CAD build for the part. Positions are in the model's coordinates, mm. Round coordinates to 2 decimals unless told otherwise and drop trailing zeros. Write each loop counter-clockwise with the first axis right and the second up, starting at its lowest first coordinate (ties: lowest second). Pieces come first, ordered by that corner, then holes. Notation, with made-up numbers: M 56,28 L 78,28 A28 cw 78,59 Z; hole C 58,75 d3. An arc over 180 degrees is marked long. Write each question's results on one line, items separated by ' | '. Start each with the question number.
```python
from build123d import *

# Parameters (mm, degrees)
CROQUIS1_W                  = 215.9
CROQUIS1_H                  = 146.05
SALIENTE_EXTRUIR1_DEPTH     = 3.1242
CROQUIS2_R                  = 1.3335
CORTAR_EXTRUIR1_DEPTH       = 131.36722652
CROQUIS9_R                  = 1.27
CORTAR_EXTRUIR6_DEPTH       = 131.36722652
CORTAR_EXTRUIR2_DEPTH       = 131.36722652
DIFERENCIAL_TRASERO_DEPTH   = 131.36722652
ENTRADA_TRANSMISION_DEPTH   = 131.36722652
CROQUIS10_R                 = 1.016
CROQUIS10_W                 = 22.606
CROQUIS10_H                 = 11.9888
CROQUIS10_W_2               = 2.032
CROQUIS10_H_2               = 5.08
SERVO_DEPTH                 = 131.36722652
CROQUIS12_R                 = 1.651
SOPORTES_BS_DEPTH           = 131.36722652
CROQUIS7_R                  = 1.5875
CROQUIS7_W                  = 11.1125
CROQUIS7_H                  = 2.9972
SOPORTE_EJE_DEPTH           = 131.36722652
CROQUIS13_R                 = 1.016
CROQUIS13_W                 = 10.922
CROQUIS13_H                 = 2.9972
CROQUIS13_W_2               = 2.9972
CROQUIS13_H_2               = 10.922
SENSORES_DE_PRESENCIA_DEPTH = 131.36722652


with BuildPart() as part:
    # Croquis1 → Saliente-Extruir1 (new body)
    with BuildSketch(Plane.XY):
        Rectangle(CROQUIS1_W, CROQUIS1_H)
    extrude(amount=SALIENTE_EXTRUIR1_DEPTH)

    # Croquis2 → Cortar-Extruir1 (cut, through all)
    with BuildSketch(Plane.XY.offset(3.1242)):
        with BuildLine():
            ThreePointArc((82.1674125, 60.7314), (81.516352882, 61.877042778), (80.1989125, 61.904002767))
            Line((80.1989125, 61.904002767), (80.1989125, 59.558797233))
            ThreePointArc((80.1989125, 59.558797233), (81.516352882, 59.585757222), (82.1674125, 60.7314))
        make_face()
        with BuildLine():
            Line((80.1989125, 59.558797233), (80.1989125, 61.904002767))
            ThreePointArc((80.1989125, 61.904002767), (79.5004125, 60.7314), (80.1989125, 59.558797233))
        make_face()
        with Locations(Location((80.8339125, -60.7314, 0), (0, 0, 180))):
            Circle(CROQUIS2_R)
    extrude(amount=-CORTAR_EXTRUIR1_DEPTH, mode=Mode.SUBTRACT)

    # Croquis9 → Cortar-Extruir6 (cut, through all)
    with BuildSketch(Plane.XY.offset(3.1242)):
        with Locations((93.5339125, 37.6809)):
            Circle(CROQUIS9_R)
        with Locations(Location((93.5339125, -37.6809, 0), (0, 0, 180))):
            Circle(CROQUIS9_R)
        with Locations((79.5639125, 37.6809)):
            Circle(CROQUIS9_R)
        with Locations((79.5639125, -37.6809)):
            Circle(CROQUIS9_R)
    extrude(amount=-CORTAR_EXTRUIR6_DEPTH, mode=Mode.SUBTRACT)

    # Croquis3 → Cortar-Extruir2 (cut, through all)
    with BuildSketch(Plane.XY.offset(3.1242)):
        with BuildLine():
            ThreePointArc((31.75, 73.025), (36.240128061, 71.165128061), (38.1, 66.675))
            Line((38.1, 66.675), (38.1, 60.648925294))
            ThreePointArc((38.1, 60.648925294), (44.483976367, 49.058906773), (56.88726875, 44.45))
            ThreePointArc((56.88726875, 44.45), (68.952768587, 48.752886462), (75.572740263, 59.719521917))
            ThreePointArc((75.572740263, 59.719521917), (75.649024122, 60.222907145), (75.6745375, 60.7314))
            ThreePointArc((75.6745375, 60.7314), (79.079726884, 65.583408163), (84.800442563, 64.030762007))
            ThreePointArc((84.800442563, 64.030762007), (101.984927744, 34.043503392), (107.95, 0))
            Line((107.95, 0), (107.95, 73.025))
            Line((107.95, 73.025), (31.75, 73.025))
        make_face()
        with BuildLine():
            Line((107.95, -73.025), (107.95, 0))
            ThreePointArc((107.95, 0), (101.984927744, -34.043503392), (84.800442563, -64.030762007))
            ThreePointArc((84.800442563, -64.030762007), (79.079726884, -65.583408163), (75.6745375, -60.7314))
            ThreePointArc((75.6745375, -60.7314), (75.649024122, -60.222907145), (75.572740263, -59.719521917))
            ThreePointArc((75.572740263, -59.719521917), (68.952768587, -48.752886462), (56.88726875, -44.45))
            ThreePointArc((56.88726875, -44.45), (44.483976367, -49.058906773), (38.1, -60.648925294))
            Line((38.1, -60.648925294), (38.1, -66.675))
            ThreePointArc((38.1, -66.675), (36.240128061, -71.165128061), (31.75, -73.025))
            Line((31.75, -73.025), (107.95, -73.025))
        make_face()
        with BuildLine():
            ThreePointArc((-107.95, 63.5), (-105.160192091, 70.235192091), (-98.425, 73.025))
            Line((-98.425, 73.025), (-107.95, 73.025))
            Line((-107.95, 73.025), (-107.95, 63.5))
        make_face()
        with BuildLine():
            Line((-107.95, -73.025), (-98.425, -73.025))
            ThreePointArc((-98.425, -73.025), (-105.160192091, -70.235192091), (-107.95, -63.5))
            Line((-107.95, -63.5), (-107.95, -73.025))
        make_face()
    extrude(amount=-CORTAR_EXTRUIR2_DEPTH, mode=Mode.SUBTRACT)

    # Croquis8 → Diferencial trasero (cut, through all)
    with BuildSketch(Plane.XY.offset(3.1242)):
        with BuildLine():
            Line((-62.484, 29.2862), (-59.944, 29.2862))
            ThreePointArc((-59.944, 29.2862), (-58.674, 28.0162), (-59.944, 26.7462))
            Line((-59.944, 26.7462), (-62.484, 26.7462))
            ThreePointArc((-62.484, 26.7462), (-63.754, 28.0162), (-62.484, 29.2862))
        make_face()
        with BuildLine():
            Line((-95.25, 55.6006), (-92.71, 55.6006))
            ThreePointArc((-92.71, 55.6006), (-91.44, 54.3306), (-92.71, 53.0606))
            Line((-92.71, 53.0606), (-95.25, 53.0606))
            ThreePointArc((-95.25, 53.0606), (-96.52, 54.3306), (-95.25, 55.6006))
        make_face()
    extrude(amount=-DIFERENCIAL_TRASERO_DEPTH, mode=Mode.SUBTRACT)

    # Croquis11 → Entrada transmision (cut, through all)
    with BuildSketch(Plane.XY.offset(3.1242)):
        with BuildLine():
            ThreePointArc((-96.8375, 73.025), (-95.984195865, 72.776166614), (-95.398394794, 72.107673453))
            Line((-95.398394794, 72.107673453), (-95.398394794, 67.0052))
            ThreePointArc((-95.398394794, 67.0052), (-94.93342681, 65.882667985), (-93.810894794, 65.4177))
            Line((-93.810894794, 65.4177), (-46.185894794, 65.4177))
            ThreePointArc((-46.185894794, 65.4177), (-45.063362779, 65.882667985), (-44.598394794, 67.0052))
            Line((-44.598394794, 67.0052), (-44.598394794, 71.4375))
            ThreePointArc((-44.598394794, 71.4375), (-44.13342681, 72.560032015), (-43.010894794, 73.025))
            Line((-43.010894794, 73.025), (-96.8375, 73.025))
        make_face()
        with BuildLine():
            Line((-96.8375, -73.025), (-43.010894794, -73.025))
            ThreePointArc((-43.010894794, -73.025), (-44.13342681, -72.560032015), (-44.598394794, -71.4375))
            Line((-44.598394794, -71.4375), (-44.598394794, -67.0052))
            ThreePointArc((-44.598394794, -67.0052), (-45.063362779, -65.882667985), (-46.185894794, -65.4177))
            Line((-46.185894794, -65.4177), (-93.810894794, -65.4177))
            ThreePointArc((-93.810894794, -65.4177), (-94.93342681, -65.882667985), (-95.398394794, -67.0052))
            Line((-95.398394794, -67.0052), (-95.398394794, -72.107673453))
            ThreePointArc((-95.398394794, -72.107673453), (-95.984195865, -72.776166614), (-96.8375, -73.025))
        make_face()
        with BuildLine():
            Line((-57.298394794, 63.8302), (-82.698394794, 63.8302))
            ThreePointArc((-82.698394794, 63.8302), (-83.259660802, 63.597716008), (-83.492144794, 63.03645))
            Line((-83.492144794, 63.03645), (-83.492144794, 52.0827))
            ThreePointArc((-83.492144794, 52.0827), (-83.724628787, 51.521433992), (-84.285894794, 51.28895))
            Line((-84.285894794, 51.28895), (-96.36125, 51.28895))
            ThreePointArc((-96.36125, 51.28895), (-96.922516008, 51.056466008), (-97.155, 50.4952))
            Line((-97.155, 50.4952), (-97.155, 30.7467))
            ThreePointArc((-97.155, 30.7467), (-96.922516008, 30.185433992), (-96.36125, 29.95295))
            Line((-96.36125, 29.95295), (-57.298394794, 29.95295))
            ThreePointArc((-57.298394794, 29.95295), (-56.737128787, 30.185433992), (-56.504644794, 30.7467))
            Line((-56.504644794, 30.7467), (-56.504644794, 63.03645))
            ThreePointArc((-56.504644794, 63.03645), (-56.737128787, 63.597716008), (-57.298394794, 63.8302))
        make_face()
    extrude(amount=-ENTRADA_TRANSMISION_DEPTH, mode=Mode.SUBTRACT)

    # Croquis10 → Servo (cut, through all)
    with BuildSketch(Plane.XY.offset(3.1242)):
        with Locations((65.1637, 0)):
            Circle(CROQUIS10_R)
        with Locations((92.6211, 0)):
            Circle(CROQUIS10_R)
        with Locations((78.8924, 0)):
            Rectangle(CROQUIS10_W, CROQUIS10_H)
        with Locations((91.2114, 0)):
            Rectangle(CROQUIS10_W_2, CROQUIS10_H_2)
    extrude(amount=-SERVO_DEPTH, mode=Mode.SUBTRACT)

    # Croquis12 → Soportes BS (cut, through all)
    with BuildSketch(Plane.XY.offset(3.1242)):
        with Locations((44.45, 41.275)):
            Circle(CROQUIS12_R)
        with Locations((-44.45, 41.275)):
            Circle(CROQUIS12_R)
        with Locations((-44.45, -41.275)):
            Circle(CROQUIS12_R)
        with Locations((44.45, -41.275)):
            Circle(CROQUIS12_R)
    extrude(amount=-SOPORTES_BS_DEPTH, mode=Mode.SUBTRACT)

    # Croquis7 → Soporte eje (cut, through all)
    with BuildSketch(Plane.XY.offset(3.1242)):
        with Locations((-80.317144794, -50.8889)):
            Circle(CROQUIS7_R)
        with Locations((-59.679644794, -50.8889)):
            Circle(CROQUIS7_R)
        with Locations((-69.998394794, -50.8889)):
            Rectangle(CROQUIS7_W, CROQUIS7_H)
    extrude(amount=-SOPORTE_EJE_DEPTH, mode=Mode.SUBTRACT)

    # Croquis13 → Sensores de presencia (cut, through all)
    with BuildSketch(Plane.XY.offset(3.1242)):
        with Locations((11.811, 68.3514)):
            Circle(CROQUIS13_R)
        with Locations(Location((-103.2764, 11.811, 0), (0, 0, 180))):
            Circle(CROQUIS13_R)
        with Locations((-103.2764, -11.811)):
            Circle(CROQUIS13_R)
        with Locations((-11.811, 68.3514)):
            Circle(CROQUIS13_R)
        with Locations(Location((-11.811, -68.3514, 0), (0, 0, 180))):
            Circle(CROQUIS13_R)
        with Locations(Location((11.811, -68.3514, 0), (0, 0, 180))):
            Circle(CROQUIS13_R)
        with Locations((98.5139, 29.972)):
            Circle(CROQUIS13_R)
        with Locations(Location((98.5139, 6.35, 0), (0, 0, 180))):
            Circle(CROQUIS13_R)
        with Locations((98.5139, -6.35)):
            Circle(CROQUIS13_R)
        with Locations(Location((98.5139, -29.972, 0), (0, 0, 180))):
            Circle(CROQUIS13_R)
        with Locations((0, 68.3514)):
            Rectangle(CROQUIS13_W, CROQUIS13_H)
        with Locations((-103.2764, 0)):
            Rectangle(CROQUIS13_W_2, CROQUIS13_H_2)
        with Locations((0, -68.3514)):
            Rectangle(CROQUIS13_W, CROQUIS13_H)
        with Locations((98.5139, 18.161)):
            Rectangle(CROQUIS13_W_2, CROQUIS13_H_2)
        with Locations((98.5139, -18.161)):
            Rectangle(CROQUIS13_W_2, CROQUIS13_H_2)
    extrude(amount=-SENSORES_DE_PRESENCIA_DEPTH, mode=Mode.SUBTRACT)


solid = part.part
```
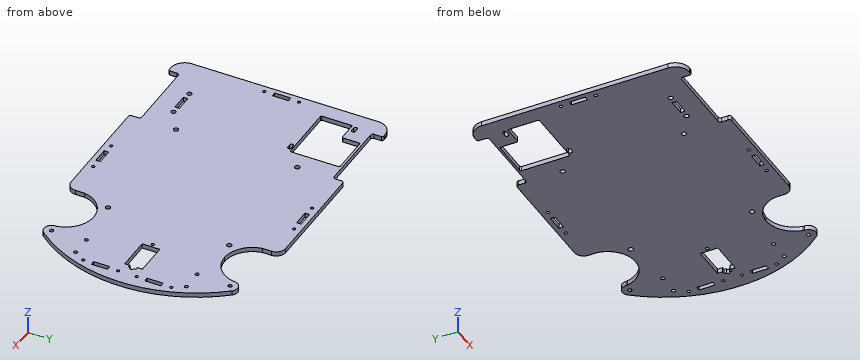
1) Drop flat-ended pins along their axis: pin 1 Ø1.3 at (x, z) = (-93.5, 1) entering from -Y; pin 2 Ø0.9 at (y, z) = (-20.5, 1) entering from +X; pin 3 Ø1.6 at (x, z) = (-74.5, 2) entering from -Y; pin 4 Ø1.2 at (x, y) = (98.51, -29.97) entering from -Z. Give the stop position or say it passes through.
2) Saw through at A-A, the plane x = 71.5. Write the cut outline in (y, z), plus the area to 3 significant figures.
3) Saw through at B-B, the plane z = 1. State how many separate pieces and enclosed holes the cut face has, plus the area to 3 significant figures.
4) Wall check: line 1 along Y through (x, z) = (-60, 2.7); line 2 along Y through (x, z) = (85, 1.3); line 3 along Y through (x, z) = (-44.45, 0.75). Give the ranges that are in metal, low to high. Write a range as from..to.
Filled sheet:
1) pin 1: stops at y = -65.45 | pin 2: stops at x = 105.92 | pin 3: stops at y = -65.42 | pin 4: passes through
2) outline: M -51.27,0 L -5.99,0 L -5.99,3.12 L -51.27,3.12 Z; M 5.99,0 L 51.27,0 L 51.27,3.12 L 5.99,3.12 Z | area: 283 mm^2
3) separate pieces: 1 | enclosed holes: 33 | area: 25,500 mm^2
4) line 1: y = -65.42..-52.44, -49.33..26.75, 29.29..29.95, 63.83..65.42 | line 2: y = -63.79..-5.99, 5.99..63.79 | line 3: y = -72.11..-42.93, -39.62..39.62, 42.93..72.11
